Input: part model. Units: mm. Frame: model coordinates. A direction names the side the tool comes from. Give positions to 0.01 mm unless a question says otherwise; leave off trailing zeros. Loops run counter-clockwise (first coordinate to the right, second up) from the corner with the lowest first, then second, coordinate; pieces in that order, holes last. Notation, with made-up numbers: (42.25, 64) -> (54.25, 64) arc R26 cw to (54.25, 96) -> close; hole circle Ø9 at (9, 62.5). An arc over 180 degrees is marked (long way). Answer in a Markdown table with one row per item. Add a question column.
```python
from build123d import *

# Parameters (mm, degrees)
EXTRUDE_1_DEPTH           = 150
EXTRUDE_1_DEPTH_BACK      = 150
SKETCH_4_R                = 2.5
CUT_EXTRUDE_4_DEPTH       = 3
SKETCH_5_W                = 52
SKETCH_5_H                = 100
CUT_EXTRUDE_5_DEPTH       = 3
SKETCH_7_R                = 1.6
SKETCH_7_R_2              = 6.5
CUT_EXTRUDE_9_DEPTH       = 185.063533313
SKETCH_6_W                = 40
SKETCH_6_H                = 200
CUT_EXTRUDE_10_DEPTH      = 10
CUT_EXTRUDE_12_DEPTH      = 4
SKETCH_12_W               = 34
SKETCH_12_H               = 110
CUT_EXTRUDE_13_DEPTH      = 4
SKETCH_14_W               = 4.2
SKETCH_14_H               = 14
CUT_EXTRUDE_14_DEPTH      = 10
SKETCH_15_R               = 2
CUT_EXTRUDE_15_DEPTH      = 26
SKETCH_17_R               = 1.5
CUT_EXTRUDE_19_DEPTH      = 10
CUT_EXTRUDE_20_DEPTH      = 10
CUT_EXTRUDE_21_DEPTH      = 31
SKETCH_22_R               = 1.5
CUT_EXTRUDE_22_DEPTH      = 31
SKETCH_23_W               = 12
SKETCH_23_H               = 87.5
EXTRUDE_3_DEPTH           = 3
CUT_EXTRUDE_23_DEPTH      = 18
CUT_EXTRUDE_24_DEPTH      = 13
CUT_EXTRUDE_24_DEPTH_BACK = 4
SKETCH_25_R               = 1.5
SKETCH_26_R               = 2
CUT_EXTRUDE_25_DEPTH      = 10
SKETCH_27_R               = 1.5
CUT_EXTRUDE_26_DEPTH      = 10
CUT_EXTRUDE_29_DEPTH      = 10
SKETCH_32_W               = 44.628479445
SKETCH_32_H               = 8.012675998
CUT_EXTRUDE_30_DEPTH      = 345
SKETCH_33_W               = 3
SKETCH_33_H               = 15
CUT_EXTRUDE_31_DEPTH      = 3


with BuildPart() as part:
    # Sketch 1 → Extrude 1 (new, two sides: drawn at the far end of the back side and taken through both)
    with BuildSketch(Plane.XY.offset(-EXTRUDE_1_DEPTH_BACK)):
        Polygon((0, 4.173281966), (0, -73.826718034), (3, -73.826718034), (3, 1.173281966), (3, 3.173281966), (5, 3.173281966), (80, 3.173281966), (80, 6.173281966), (2, 6.173281966), (0, 6.173281966), align=None)
    extrude(amount=EXTRUDE_1_DEPTH + EXTRUDE_1_DEPTH_BACK)

    # Sketch 4 → Cut-Extrude 4 (cut)
    with BuildSketch(Plane(origin=(0, 6.173281966, 0), x_dir=(1, 0, 0), z_dir=(0, 1, 0))):
        with Locations(Location((11.5, -72.5, 0), (0, 0, 180))):
            Circle(SKETCH_4_R)
        with Locations(Location((11.5, -127.5, 0), (0, 0, 180))):
            Circle(SKETCH_4_R)
    extrude(amount=-CUT_EXTRUDE_4_DEPTH, mode=Mode.SUBTRACT)

    # Sketch 5 → Cut-Extrude 5 (cut)
    with BuildSketch(Plane(origin=(0, 6.173281966, 0), x_dir=(1, 0, 0), z_dir=(0, 1, 0))):
        with Locations((54, -100)):
            Rectangle(SKETCH_5_W, SKETCH_5_H)
    extrude(amount=-CUT_EXTRUDE_5_DEPTH, mode=Mode.SUBTRACT)

    # Sketch 7 → Cut-Extrude 9 (cut, through all)
    with BuildSketch(Plane(origin=(3, 0, 0), x_dir=(0, 0, -1), z_dir=(1, 0, 0))):
        with Locations(Location((-54.5, -43.826718034, 0), (0, 0, 90))):
            Circle(SKETCH_7_R)
        with Locations(Location((-62.25, -30.403324275, 0), (0, 0, 90))):
            Circle(SKETCH_7_R)
        with Locations(Location((-62.25, -57.250111793, 0), (0, 0, 90))):
            Circle(SKETCH_7_R)
        with Locations(Location((-77.75, -30.403324275, 0), (0, 0, 90))):
            Circle(SKETCH_7_R)
        with Locations(Location((-77.75, -57.250111793, 0), (0, 0, 90))):
            Circle(SKETCH_7_R)
        with Locations(Location((-85.5, -43.826718034, 0), (0, 0, 90))):
            Circle(SKETCH_7_R)
        with Locations(Location((115.5, -43.826718034, 0), (0, 0, 90))):
            Circle(SKETCH_7_R)
        with Locations(Location((107.75, -30.403324275, 0), (0, 0, 90))):
            Circle(SKETCH_7_R)
        with Locations(Location((107.75, -57.250111793, 0), (0, 0, 90))):
            Circle(SKETCH_7_R)
        with Locations(Location((92.25, -30.403324275, 0), (0, 0, 90))):
            Circle(SKETCH_7_R)
        with Locations(Location((92.25, -57.250111793, 0), (0, 0, 90))):
            Circle(SKETCH_7_R)
        with Locations(Location((84.5, -43.826718034, 0), (0, 0, 90))):
            Circle(SKETCH_7_R)
        with Locations(Location((-70, -50.826718034, 0), (0, 0, 90))):
            Circle(SKETCH_7_R_2)
        with Locations(Location((100, -50.826718034, 0), (0, 0, 90))):
            Circle(SKETCH_7_R_2)
    extrude(amount=-CUT_EXTRUDE_9_DEPTH, mode=Mode.SUBTRACT)

    # Sketch 6 → Cut-Extrude 10 (cut)
    with BuildSketch(Plane(origin=(0, 6.173281966, 0), x_dir=(1, 0, 0), z_dir=(0, 1, 0))):
        with Locations((60, 50)):
            Rectangle(SKETCH_6_W, SKETCH_6_H)
    extrude(amount=-CUT_EXTRUDE_10_DEPTH, mode=Mode.SUBTRACT)

    # Sketch 11 → Cut-Extrude 12 (cut)
    with BuildSketch(Plane.ZY):
        Polygon((-128.345117246, -73.826718034), (-150, -73.826718034), (-150, 3.173281966), align=None)
    extrude(amount=-CUT_EXTRUDE_12_DEPTH, mode=Mode.SUBTRACT)

    # Sketch 12 → Cut-Extrude 13 (cut)
    with BuildSketch(Plane(origin=(0, 6.173281966, 0), x_dir=(1, 0, 0), z_dir=(0, 1, 0))):
        with Locations((23, 95)):
            Rectangle(SKETCH_12_W, SKETCH_12_H)
    extrude(amount=-CUT_EXTRUDE_13_DEPTH, mode=Mode.SUBTRACT)

    # Sketch 14 → Cut-Extrude 14 (cut)
    with BuildSketch(Plane.XZ.offset(-3.173281966)):
        with Locations((5.1, -103)):
            Rectangle(SKETCH_14_W, SKETCH_14_H)
    extrude(amount=-CUT_EXTRUDE_14_DEPTH, mode=Mode.SUBTRACT)

    # Sketch 15 → Cut-Extrude 15 (cut)
    with BuildSketch(Plane(origin=(0, 6.173281966, 0), x_dir=(1, 0, 0), z_dir=(0, 1, 0))):
        with Locations(Location((32, -4.5, 0), (0, 0, 270))):
            Circle(SKETCH_15_R)
    extrude(amount=-CUT_EXTRUDE_15_DEPTH, mode=Mode.SUBTRACT)

    # Sketch 17 → Cut-Extrude 19 (cut)
    with BuildSketch(Plane.XZ.offset(-3.173281966)):
        with Locations((23.690733746, 113.5)):
            Circle(SKETCH_17_R)
    extrude(amount=-CUT_EXTRUDE_19_DEPTH, mode=Mode.SUBTRACT)

    # Sketch 18 → Cut-Extrude 20 (cut)
    with BuildSketch(Plane.ZY):
        Polygon((150, -73.826718034), (118.550084008, -73.826718034), (150, 0), align=None)
    extrude(amount=-CUT_EXTRUDE_20_DEPTH, mode=Mode.SUBTRACT)

    # Sketch 21 → Cut-Extrude 21 (cut)
    with BuildSketch(Plane.ZY):
        Polygon((118.550084008, -73.826718034), (150, 0), (150, 6.173281966), (137.5, 6.173281966), (132.072189672, -6.568164552), (98.550084008, -73.826718034), align=None)
    extrude(amount=-CUT_EXTRUDE_21_DEPTH, mode=Mode.SUBTRACT)

    # Sketch 22 → Cut-Extrude 22 (cut)
    with BuildSketch(Plane.ZY):
        with Locations(Location((-106, 3.173281966, 0), (0, 0, 270))):
            Circle(SKETCH_22_R)
        with Locations(Location((-100, 3.173281966, 0), (0, 0, 270))):
            Circle(SKETCH_22_R)
        with Locations(Location((-106, -1.826718034, 0), (0, 0, 270))):
            Circle(SKETCH_22_R)
        with Locations(Location((-100, -1.826718034, 0), (0, 0, 270))):
            Circle(SKETCH_22_R)
    extrude(amount=-CUT_EXTRUDE_22_DEPTH, mode=Mode.SUBTRACT)

    # Sketch 23 → Extrude 3 (add)
    with BuildSketch(Plane(origin=(0, 6.173281966, 0), x_dir=(1, 0, 0), z_dir=(0, 1, 0))):
        with Locations((34, -93.75)):
            Rectangle(SKETCH_23_W, SKETCH_23_H)
    extrude(amount=-EXTRUDE_3_DEPTH)

    # Sketch 24 → Cut-Extrude 23 (cut)
    with BuildSketch(Plane.ZY.offset(-28)):
        Polygon((137.5, 6.173281966), (137.5, 3.173281966), (136.222010805, 3.173281966), align=None)
    extrude(amount=-CUT_EXTRUDE_23_DEPTH, mode=Mode.SUBTRACT)

    # Sketch 25 → Cut-Extrude 24 (cut, two sides: drawn at the far end of the back side and taken through both)
    with BuildSketch(Plane(origin=(0, 6.173281966, 0), x_dir=(1, 0, 0), z_dir=(0, 1, 0)).offset(-CUT_EXTRUDE_24_DEPTH_BACK)):
        with Locations((32, -61)):
            Circle(SKETCH_25_R)
    extrude(amount=CUT_EXTRUDE_24_DEPTH + CUT_EXTRUDE_24_DEPTH_BACK, mode=Mode.SUBTRACT)

    # Sketch 26 → Cut-Extrude 25 (cut)
    with BuildSketch(Plane.XZ.offset(-3.173281966)):
        with Locations((32, -25.5)):
            Circle(SKETCH_26_R)
    extrude(amount=-CUT_EXTRUDE_25_DEPTH, mode=Mode.SUBTRACT)

    # Sketch 27 → Cut-Extrude 26 (cut)
    with BuildSketch(Plane.XZ.offset(-3.173281966)):
        with Locations((23.690733746, 123.5)):
            Circle(SKETCH_27_R)
    extrude(amount=-CUT_EXTRUDE_26_DEPTH, mode=Mode.SUBTRACT)

    # Sketch 31 → Cut-Extrude 29 (cut)
    with BuildSketch(Plane(origin=(3, 0, 0), x_dir=(0, 0, -1), z_dir=(1, 0, 0))):
        Polygon((-38.550084008, -73.826718034), (-10.102483381, -23.826718034), (39.897516619, -23.826718034), (68.345117246, -73.826718034), align=None)
    extrude(amount=-CUT_EXTRUDE_29_DEPTH, mode=Mode.SUBTRACT)

    # Sketch 32 → Cut-Extrude 30 (cut)
    with BuildSketch(Plane(origin=(0, 0, -150), x_dir=(-1, 0, 0), z_dir=(0, 0, -1))):
        with Locations((-25.314239723, 7.179619965)):
            Rectangle(SKETCH_32_W, SKETCH_32_H)
    extrude(amount=-CUT_EXTRUDE_30_DEPTH, mode=Mode.SUBTRACT)

    # Sketch 33 → Cut-Extrude 31 (cut)
    with BuildSketch(Plane(origin=(0, 6.173281966, 0), x_dir=(1, 0, 0), z_dir=(0, 1, 0))):
        with Locations((1.5, 32.5)):
            Rectangle(SKETCH_33_W, SKETCH_33_H)
        with Locations((1.5, -57.5)):
            Rectangle(SKETCH_33_W, SKETCH_33_H)
    extrude(amount=-CUT_EXTRUDE_31_DEPTH, mode=Mode.SUBTRACT)


solid = part.part
```
1) Section D-D on z = -35.5. Output: boundary loops of the cut face in (x, y), and give its area (3 significant figures).
2) Reachability of faces 1 (the face through (1.521, -49.177, 24.525)), 2 (the face through (1.521, -52.236, 63.655)) from +Z, -Z, +X, -X, +Y, -Y: full face, straight path, thin tool, end or side. Return the list, or none.
3) Pin query (flat end, axial travel): pin 1 (5 mm diameter, centred on y = -43.83, z = 54.5, fed in from -X); pin 2 (0.9 mm diameter, centred on x = 1, y = 4, fed in from +Z); pin 3 (1.5 mm diameter, centred on x = 0.5, y = -3, fed in from +Z); pin 4 (0.9 mm diameter, centred on x = 1.5, z = -9.5, fed in from -Y). Return the tip coordinate at first contact, or that it passes through.
4) Section C-C on x = 2. State how many separate pieces and enclosed holes the cut face has, and give its area (3 significant figures).
5) Section A-A on z = 70. Output: boundary loops of the cut face in (x, y), and give its area (3 significant figures).
6) Pull-direction query (Y, two-part tool) for faces 3 (the face through (1.479, -39.727, 115.546)), 4 (the face through (1.521, -52.236, -106.345)), 5 (the face through (3, -17, -8)); classes: +Y half, -Y half, draft (parallel to the pull), parting line (faces both ways), or undercut.
7) Section B-B on y = -63. Output: boundary loops of the cut face in (x, z).
8) Material intervals for line 1 along Y through (x, z) = (1.9, -92.25); line 2 along Y through (x, z) = (2.4, 85.5); line 3 along Z through (x, y) = (2.65, -29), sorted ascending.
Working result:
| question | item | result |
|---|---|---|
| 1 | outline | (0, -23.83) -> (3, -23.83) -> (3, 3.17) -> (0, 3.17) -> close |
| 1 | area | 81.0 mm2 |
| 2 | face 1 | +X, -X, -Y |
| 2 | face 2 | +X, -X |
| 3 | pin 1 | stops at x = 0 |
| 3 | pin 2 | stops at z = 136.77 |
| 3 | pin 3 | stops at z = 133.91 |
| 3 | pin 4 | stops at y = -23.83 |
| 4 | separate pieces | 1 |
| 4 | enclosed holes | 18 |
| 4 | area | 16,200 mm2 |
| 5 | outline | (0, -73.83) -> (3, -73.83) -> (3, -57.33) -> (0, -57.33) -> close; (0, -44.33) -> (3, -44.33) -> (3, 6.17) -> (0, 6.17) -> close |
| 5 | area | 201 mm2 |
| 6 | face 3 | -Y half |
| 6 | face 4 | undercut |
| 6 | face 5 | draft |
| 7 | outline | (0, -131.39) -> (3, -131.39) -> (3, -62.19) -> (0, -62.19) -> close; (0, 32.39) -> (3, 32.39) -> (3, 103.95) -> (0, 103.95) -> close |
| 8 | line 1 | y = -73.83 to -58.85, -55.65 to -32, -28.8 to 6.17 |
| 8 | line 2 | y = -73.83 to -45.43, -42.23 to 6.17 |
| 8 | line 3 | z = -140.95 to -108.52, -106.98 to -93.02, -91.48 to -42.84, 13.05 to 61.48, 63.02 to 76.98, 78.52 to 120.89 |
